The listing builds one solid part. Answer for the finished solid, in the listing's coordinates (mm). Give positions to 0.01 mm unless a question says otherwise; leave off trailing zeros. Order: outer loops, then holes, each group sorted by start corner. A loop starts at its lowest first (then second) coordinate and runs counter-clockwise, first axis right, second up. Notation, with made-up numbers: (-5, 89) - (43, 89) arc R26 cw to (43, 107) - close; hole circle Ø8 at (71.25, -22). An arc over 180 degrees is marked (long way). Use a Markdown table: item, result. Add a question column.
1) Find section B-B, the plane z = 42. Determine the outline of the cut face in (x, y).
2) Find section D-D, the plane z = 8. Determine the outline of the cut face in (x, y).
3) Find section A-A, the plane y = 29.5. Determine the outline of the cut face in (x, z).
4) The mould has two halves that part along Z. Classify faces 1 (the face through (1, 46, 31)), 2 (the face through (1, 23, 0)), 3 (the face through (1.52, 42.18, 40.89)): released by +Z, released by -Z, zero draft, split by the parting line, or undercut.
5) A flat-ended cylindrical pin translates along its axis: pin 1 (3 mm diameter, centred on y = 29.5, z = 8, fed in from +X). Find the tip coordinate at first contact, or state that the pin passes through.
6) Straight lines are drawn through the part: line 1 (Z direction, x = 2.2, y = 29.5); line 2 (Z direction, x = 1.6, y = 16.5); line 3 (Y direction, x = 2.8, z = 9.5). For each, find the intervals that lie inside material, in ascending order.
7) Find section C-C, the plane x = 0.55. Determine the outline of the cut face in (y, z), plus the area to 3 significant figures.
from build123d import *

# Parameters (mm, degrees)
F0_W     = 46
F0_H     = 63
F1_DEPTH = 3
F2_W     = 46
F2_H     = 63
F2_R     = 2.4
F2_R_2   = 2.9
F3_DEPTH = 3.001


with BuildPart() as f1:
    # F0 (on Right) → F1 (new body)
    with BuildSketch(Plane.YZ):
        with Locations((23, 31.5)):
            Rectangle(F0_W, F0_H)
    extrude(amount=F1_DEPTH)

    # F2 (on face) → F3 (intersect, through all)
    with BuildSketch(Plane.YZ.offset(3)):
        with Locations((23, 31.5)):
            Rectangle(F2_W, F2_H)
        with Locations((12.5, 8)):
            Circle(F2_R, mode=Mode.SUBTRACT)
        with Locations((29.5, 8)):
            Circle(F2_R, mode=Mode.SUBTRACT)
        with Locations((16.5, 42)):
            Circle(F2_R_2, mode=Mode.SUBTRACT)
        with Locations((39.5, 42)):
            Circle(F2_R_2, mode=Mode.SUBTRACT)
    extrude(amount=-F3_DEPTH, mode=Mode.INTERSECT)


solid = f1.part
The answers:
| question | item | result |
|---|---|---|
| 1 | outline | (0, 0) - (3, 0) - (3, 13.6) - (0, 13.6) - close; (0, 19.4) - (3, 19.4) - (3, 36.6) - (0, 36.6) - close; (0, 42.4) - (3, 42.4) - (3, 46) - (0, 46) - close |
| 2 | outline | (0, 0) - (3, 0) - (3, 10.1) - (0, 10.1) - close; (0, 14.9) - (3, 14.9) - (3, 27.1) - (0, 27.1) - close; (0, 31.9) - (3, 31.9) - (3, 46) - (0, 46) - close |
| 3 | outline | (0, 0) - (3, 0) - (3, 5.6) - (0, 5.6) - close; (0, 10.4) - (3, 10.4) - (3, 63) - (0, 63) - close |
| 4 | face 1 | zero draft |
| 4 | face 2 | released by -Z |
| 4 | face 3 | undercut |
| 5 | pin 1 | through |
| 6 | line 1 | 0 to 5.6, 10.4 to 63 |
| 6 | line 2 | 0 to 39.1, 44.9 to 63 |
| 6 | line 3 | 0 to 10.63, 14.37 to 27.63, 31.37 to 46 |
| 7 | outline | (0, 0) - (46, 0) - (46, 63) - (0, 63) - close; hole circle Ø4.8 at (12.5, 8); hole circle Ø5.8 at (16.5, 42); hole circle Ø4.8 at (29.5, 8); hole circle Ø5.8 at (39.5, 42) |
| 7 | area | 2,810 mm2 |
